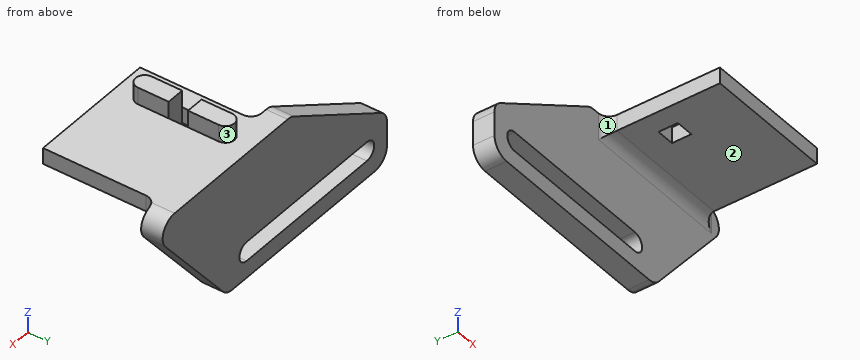
Autodesk Inventor part; units mm, degrees
ref_plane "YZ Plane" through (0, 0, 0) normal (1, 0, 0) x (0, 1, 0)
ref_plane "XZ Plane" through (0, 0, 0) normal (0, 1, 0) x (-1, 0, 0)
ref_plane "XY Plane" through (0, 0, 0) normal (0, 0, 1) x (1, 0, 0)
sketch "Sketch1" plane through (0, 0, 0) normal (0, 1, 0) x (-1, 0, 0)
  line L0 (0, 0) -> (-42.7482, 0)
  line L1 (-42.7482, 0) -> (-42.7482, -12.7)
  line L2 (-42.7482, -12.7) -> (0, -12.7)
  line L3 (0, -12.7) -> (0, 0)
  line L4 (0, -6.35) -> (-42.7482, -6.35)
  circle A0 centre (-2.286, -6.35) radius 2.286
  circle A1 centre (-40.4622, -6.35) radius 2.286
  line L5 (0, 0) -> (4.064, 0)
  line L6 (4.064, 0) -> (4.064, -12.7)
  line L7 (4.064, -12.7) -> (0, -12.7)
  line L8 (0, -12.7) -> (0, 0)
  line L9 (-42.7482, 0) -> (-46.8122, 0)
  line L10 (-46.8122, 0) -> (-46.8122, -12.7)
  line L11 (-46.8122, -12.7) -> (-42.7482, -12.7)
  line L12 (-42.7482, -12.7) -> (-42.7482, 0)
  line L13 (-2.286, -4.064) -> (-40.4622, -4.064)
  line L14 (-2.286, -8.636) -> (-40.4622, -8.636)
  dimension "d0" = 12.7
  dimension "d1" = 42.7482
  dimension "d2" = 4.572
  dimension "d3" = 4.572
  dimension "d4" = 2.286
  dimension "d5" = 2.286
  dimension "d6" = 4.064
  dimension "d7" = 4.064
extrude "Extrusion1" add sketch "Sketch1" along normal blind 5.08 contours L3 A0 L13 A1 L1 L0 | L5 L6 L7 L3 | L1 L11 L10 L9 | L3 L2 L1 A1 L14 A0
sketch "Sketch2" plane through (0, 5.08, 0) normal (0, 1, 0) x (1, 0, 0)
  line L0 (-4.064, 12.7) -> (-4.064, 0)
  line L1 (-4.064, 0) -> (46.8122, 0)
  line L2 (46.8122, 0) -> (46.8122, -17.272)
  line L3 (46.8122, -17.272) -> (-4.064, -17.272)
  line L4 (-4.064, -17.272) -> (-4.064, 0)
  point P0 (0, 0)
  point P1 (46.8122, -8.636)
  dimension "d10" = 50.8762
  dimension "d11" = 17.272
extrude "Extrusion2" add sketch "Sketch2" against normal blind 5.08
sketch "Sketch9" plane through (-4.064, 5.08, 17.272) normal (0, 0, 1) x (1, 0, 0)
  line L0 (66.2305, -31.9278) -> (66.2305, -10.0838)
  line L1 (66.2305, -31.9278) -> (35.4457, -31.9278)
  line L2 (35.4457, -10.0838) -> (35.4457, -31.9278)
  line L3 (44.7294, -25.4988) -> (44.7294, -18.2598)
  arc A0 (40.4492, -25.4988) -> (44.7294, -25.4988) centre (42.5893, -25.4988) ccw
  line L4 (40.4492, -18.2598) -> (40.4492, -25.4988)
  line L5 (44.7294, -13.6878) -> (44.7294, -18.2598)
  line L6 (40.4492, -18.2598) -> (40.4492, -13.6878)
  line L7 (40.4492, -13.6878) -> (40.4492, -6.4488)
  arc A1 (44.7294, -6.4488) -> (40.4492, -6.4488) centre (42.5893, -6.4488) ccw
  line L8 (44.7294, -6.4488) -> (44.7294, -13.6878)
  line L9 (40.4492, -13.6878) -> (44.7294, -13.6878)
  line L10 (44.7294, -18.2598) -> (40.4492, -18.2598)
  arc A2 (71.2343, -5.08) -> (66.2305, -10.0838) centre (71.2343, -10.0838) ccw
  arc A3 (35.4457, -10.0838) -> (30.4419, -5.08) centre (30.4419, -10.0838) ccw
  line L11 (40.8305, -31.9278) -> (66.2305, -31.9278)
  line L12 (29.464, -5.08) -> (71.2343, -5.08)
  line L13 (35.4457, -10.0838) -> (35.4457, -5.08)
  line L14 (66.2305, -10.0838) -> (66.2305, -5.08)
  point P0 (40.9442, -5.08)
  point P1 (30.4419, -5.08)
  point P2 (44.2344, -5.08)
  dimension "d43" = 25.4
extrude "Extrusion7" add sketch "Sketch9" against normal blind 3.81 contours L1 L2 L13 L12 A1 L7 L6 L4 A0 L3 L5 L8 L14 L0 | L12 A1 | A1 L8 L9 L7 L12 | L3 A0 L4 L10
extrude "Extrusion8" add sketch "Sketch9" along normal blind 4.0132 contours L12 A1 | A1 L8 L9 L7 L12 | L3 A0 L4 L10
sketch "Sketch10" plane through (46.8122, 0, 17.272) normal (0, 1, 0) x (1, 0, 0)
  line L0 (15.3543, 5.08) -> (20.3581, 5.08)
  line L1 (0, 0) -> (0, 29.972)
  line L2 (0, 29.972) -> (20.3581, 5.08)
  line L3 (-15.4305, 0) -> (-20.4343, 0)
  line L4 (-20.4343, 0) -> (-50.8762, 18.288)
  line L5 (-50.8762, 29.972) -> (-50.8762, 0)
  line L6 (0, 29.972) -> (-0.0381, 3.81)
  line L7 (15.3543, 3.81) -> (-15.4305, 3.81)
  line L8 (0, 0) -> (20.3581, 0)
  line L9 (20.3581, 0) -> (20.3581, 5.08)
  line L10 (20.3581, 5.08) -> (0, 5.08)
  line L11 (0, 5.08) -> (0, 0)
  line L12 (-50.8762, 29.972) -> (-50.8762, 0)
  line L13 (-50.8762, 18.288) -> (-50.8762, 0)
  line L14 (-50.8762, 0) -> (-20.4343, 0)
  point P0 (-46.8122, 17.272)
extrude "Extrusion9" add sketch "Sketch10" along normal blind 5.08 contours L10 L1 L2 L0 | L0 L9 L8 L1 L10
extrude "Extrusion10" cut sketch "Sketch10" along normal blind 5.08 contours L14 L5 L4
fillet "Fillet4" radius 3.81 6 edges at (46.8122, 2.54, -12.7) (-4.064, 2.54, -12.7) (-4.064, 2.54, -1.016) (26.3779, 2.54, 17.272) (67.1703, 2.54, 12.192) (67.1703, 2.54, 17.272)
fillet "Fillet5" radius 2.54 3 edges at (62.1665, 0, 15.367) (46.7741, 0, 13.462) (31.3817, 0, 15.367)
properties part number "Limit Switch Mount"
Can you work these out from the model? Positions are in its coordinate system, mm. Face numbers are marked on the shaded views. A direction names the side the tool comes from. Round coordinates to 2 decimals unless told otherwise and drop trailing zeros. Loops run counter-clockwise (first coordinate to the right, second up) from the corner with the lowest first, then second, coordinate; pieces in that order, holes last. Notation, with made-up numbers: M -3.75,14.5 L 23.25,14.5 A16 cw 23.25,34.5 Z; hole C -37,-2 d6. An arc over 180 degrees is marked long. Answer in a Markdown table with one row per item.
1. I'm going to push flat-ended pins straight in: pin 1 Ø2 at (y, z) = (-5.5, 19.5) entering from +X; pin 2 Ø10 at (x, y) = (26, -1) entering from +Z; pin 3 Ø3 at (y, z) = (-9.5, 15) entering from +X. Where does each tip first touch, or does it pass through?
Established:
| item | result |
|---|---|
| pin 1 | x = 40.67 |
| pin 2 | z = 17.27 |
| pin 3 | x = 62.17 |
2. If we section it at A-A, the plane x = 9.5: Please give me the cut outline in (y, z), plus the area to 3 significant figures.
Established:
| item | result |
|---|---|
| outline | M 0,-12.7 L 5.08,-12.7 L 5.08,-8.64 L 0,-8.64 Z; M 0,-4.06 L 5.08,-4.06 L 5.08,7.13 L 0,7.13 Z |
| area | 77.5 mm² |
3. If we section it at C-C, the plane z = -6.35: Please give me the cut outline in (x, y).
Established:
| item | result |
|---|---|
| outline | M -4.06,0 L 0,0 L 0,5.08 L -4.06,5.08 Z; M 42.75,0 L 52.01,0 L 52.01,5.08 L 42.75,5.08 Z |
4. If we section it at D-D, the plane x = 51: Please give me the cut outline in (y, z).
Established:
| item | result |
|---|---|
| outline | M -26.85,13.46 L -2.54,13.46 A2.54 cw 0,10.92 L 0,-7.58 L 5.08,-7.58 L 5.08,17.27 L -26.85,17.27 Z |
5. Please list where these lines run through material, in increasing order: line 1 (X direction, y = -10, z = 15.5); line 2 (Z direction, x = 43.5, y = -4); line 3 (X direction, y = -14.5, z = 17). Write a range as from..to.
Established:
| item | result |
|---|---|
| line 1 | 31.38..36.39, 40.67..62.17 |
| line 2 | 13.46..17.27 |
| line 3 | 31.38..62.17 |
6. If we section it at B-B, the plane y = -16: Please give me the cut outline in (x, z).
Established:
| item | result |
|---|---|
| outline | M 31.38,13.46 L 62.17,13.46 L 62.17,17.27 L 40.67,17.27 L 40.67,21.29 L 36.39,21.29 L 36.39,17.27 L 31.38,17.27 Z |
7. On a 3-axis mill with a long thin cutter (end or side, diameter ignored), from which of +Z, -Z, +X, -X, +Y, -Y can I reach the whole of each face in a straight line? I mean the marked faces 1, 2 and 3. Say none if no direction works.
Established:
| item | result |
|---|---|
| face 1 | +Z, -Z, -X, -Y |
| face 2 | -Z, +X, -X, -Y |
| face 3 | +Z, +Y |
